Print and shaded views of the part. All mm, measured from the part's lowest x, y and z. Round coordinates to 2 decimals unless told otherwise and drop trailing zeros. Write each loop counter-clockwise with the first axis right and the second up, starting at its lowest first coordinate (ties: lowest second). Pieces come first, ordered by that corner, then holes. Notation, with made-up numbers: (19.5, 67) -> (42.5, 67) arc R19 ccw to (42.5, 99) -> close; hole circle Ø9 at (20, 39). An arc over 180 degrees is marked (long way). Return JSON: item names as keys, results as strings. Group by question number.
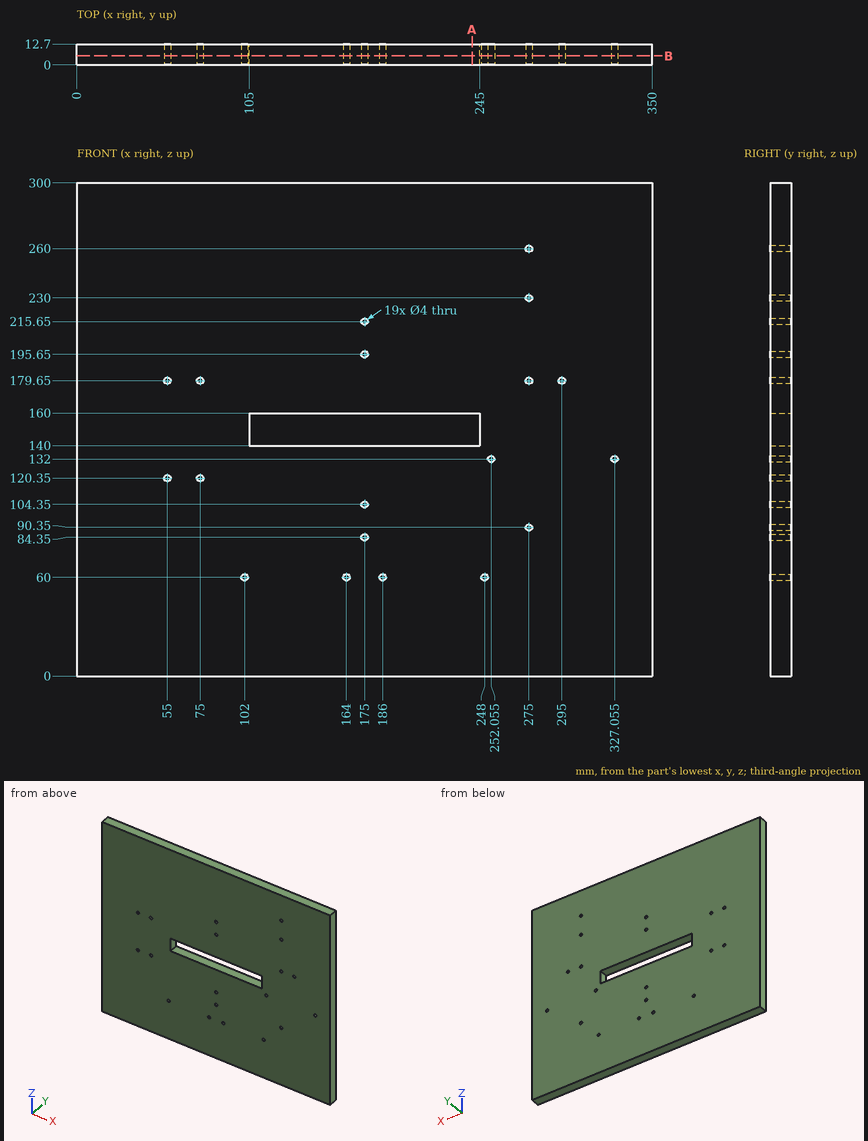
Item 1: Cut at B-B (y = 5.5). State how many separate pieces and enclosed holes the cut face has, then the cut area to 3 significant figures.
Item 2: Wall check: L1, parallel to Z at x = 275, y = 5; L2, parallel to Z at x = 275.5, y = 4.25; L3, parallel to X at y = 3.5, z = 60. Give the ranges that are in metal, low to high.
Item 3: Cut at A-A (x = 240.5). Write the cut outline in (y, z).
Item 4: Flat gauge pin, fed straight in: P1, Ø6.5, axis at x = 166.5, y = 6.5, coming from the -Z side. Where does the tip first touch, or does it go through?
Checks:
{
 "1": {"separate pieces": "1", "enclosed holes": "20", "area": "102,000 mm2"},
 "2": {"L1": "z = 0 to 88.35, 92.35 to 177.65, 181.65 to 228, 232 to 258, 262 to 300", "L2": "z = 0 to 88.41, 92.29 to 177.71, 181.59 to 228.06, 231.94 to 258.06, 261.94 to 300", "L3": "x = 0 to 100, 104 to 162, 166 to 184, 188 to 246, 250 to 350"},
 "3": {"outline": "(0, 0) -> (12.7, 0) -> (12.7, 140) -> (0, 140) -> close; (0, 160) -> (12.7, 160) -> (12.7, 300) -> (0, 300) -> close"},
 "4": {"P1": "stops at z = 0"}
}
